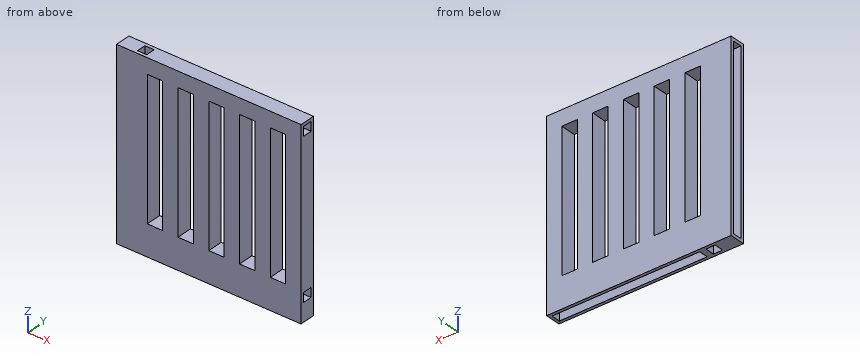
from build123d import *

# Parameters (mm, degrees)
SKETCH3_W           = 152.4
SKETCH3_H           = 152.4
BOSS_EXTRUDE1_DEPTH = 12.7
SKETCH5_W           = 147.32
SKETCH5_H           = 7.62
CUT_EXTRUDE1_DEPTH  = 12.7
SKETCH6_W           = 12.7
SKETCH6_H           = 127
CUT_EXTRUDE3_DEPTH  = 12.7
SKETCH8_W           = 7.62
SKETCH8_H           = 7.62
CUT_EXTRUDE4_DEPTH  = 25.4
SKETCH9_W           = 7.62
SKETCH9_H           = 7.62
CUT_EXTRUDE5_DEPTH  = 25.4
SKETCH10_W          = 7.508888552
SKETCH10_H          = 7.62
CUT_EXTRUDE6_DEPTH  = 25.4
SKETCH11_W          = 7.62
SKETCH11_H          = 7.62
BOSS_EXTRUDE2_DEPTH = 25.4
SKETCH12_W          = 127.135461675
SKETCH12_H          = 12.7
BOSS_EXTRUDE3_DEPTH = 25.4
SKETCH14_W          = 121.92
SKETCH14_H          = 7.62
CUT_EXTRUDE7_DEPTH  = 12.7
SKETCH15_W          = 7.62
SKETCH15_H          = 7.62
CUT_EXTRUDE9_DEPTH  = 25.4


with BuildPart() as part:
    # Sketch3 → Boss-Extrude1 (new body)
    with BuildSketch(Plane(origin=(0, 0, 0), x_dir=(1, 0, 0), z_dir=(0, 1, 0))):
        with Locations((-76.2, 76.2)):
            Rectangle(SKETCH3_W, SKETCH3_H)
    extrude(amount=BOSS_EXTRUDE1_DEPTH)

    # Sketch5 → Cut-Extrude1 (cut)
    with BuildSketch(Plane.ZY.offset(152.4)):
        with Locations((-76.2, 6.35)):
            Rectangle(SKETCH5_W, SKETCH5_H)
    extrude(amount=-CUT_EXTRUDE1_DEPTH, mode=Mode.SUBTRACT)

    # Sketch6 → Cut-Extrude3 (cut)
    with BuildSketch(Plane(origin=(0, 12.7, 0), x_dir=(1, 0, 0), z_dir=(0, 1, 0))):
        with Locations((-120.65, 76.2)):
            Rectangle(SKETCH6_W, SKETCH6_H)
        with Locations((-95.25, 76.2)):
            Rectangle(SKETCH6_W, SKETCH6_H)
        with Locations((-69.85, 76.2)):
            Rectangle(SKETCH6_W, SKETCH6_H)
        with Locations((-44.45, 76.2)):
            Rectangle(SKETCH6_W, SKETCH6_H)
        with Locations((-19.05, 76.2)):
            Rectangle(SKETCH6_W, SKETCH6_H)
    extrude(amount=-CUT_EXTRUDE3_DEPTH, mode=Mode.SUBTRACT)

    # Sketch8 → Cut-Extrude4 (cut)
    with BuildSketch(Plane(origin=(0, 0, 0), x_dir=(0, 0, -1), z_dir=(1, 0, 0))):
        with Locations((146.05, 6.35)):
            Rectangle(SKETCH8_W, SKETCH8_H)
        with Locations((6.35, 6.35)):
            Rectangle(SKETCH8_W, SKETCH8_H)
    extrude(amount=-CUT_EXTRUDE4_DEPTH, mode=Mode.SUBTRACT)

    # Sketch9 → Cut-Extrude5 (cut)
    with BuildSketch(Plane.XY):
        with Locations((-133.35, 6.35)):
            Rectangle(SKETCH9_W, SKETCH9_H)
    extrude(amount=-CUT_EXTRUDE5_DEPTH, mode=Mode.SUBTRACT)

    # Sketch10 → Cut-Extrude6 (cut)
    with BuildSketch(Plane(origin=(0, 0, -152.4), x_dir=(-1, 0, 0), z_dir=(0, 0, -1))):
        with Locations((133.405555724, 6.35)):
            Rectangle(SKETCH10_W, SKETCH10_H)
    extrude(amount=-CUT_EXTRUDE6_DEPTH, mode=Mode.SUBTRACT)

    # Sketch11 → Boss-Extrude2 (add)
    with BuildSketch(Plane(origin=(-25.4, 0, 0), x_dir=(0, 0, -1), z_dir=(1, 0, 0))):
        with Locations((146.05, 6.35)):
            Rectangle(SKETCH11_W, SKETCH11_H)
    extrude(amount=BOSS_EXTRUDE2_DEPTH)

    # Sketch12 → Boss-Extrude3 (add)
    with BuildSketch(Plane(origin=(0, 0, -152.4), x_dir=(-1, 0, 0), z_dir=(0, 0, -1))):
        with Locations((63.567730838, 6.35)):
            Rectangle(SKETCH12_W, SKETCH12_H)
    extrude(amount=-BOSS_EXTRUDE3_DEPTH)

    # Sketch14 → Cut-Extrude7 (cut)
    with BuildSketch(Plane(origin=(0, 0, -152.4), x_dir=(-1, 0, 0), z_dir=(0, 0, -1))):
        with Locations((63.5, 6.35)):
            Rectangle(SKETCH14_W, SKETCH14_H)
    extrude(amount=-CUT_EXTRUDE7_DEPTH, mode=Mode.SUBTRACT)

    # Sketch15 → Cut-Extrude9 (cut)
    with BuildSketch(Plane(origin=(0, 0, 0), x_dir=(0, 0, -1), z_dir=(1, 0, 0))):
        with Locations((133.35, 6.35)):
            Rectangle(SKETCH15_W, SKETCH15_H)
    extrude(amount=-CUT_EXTRUDE9_DEPTH, mode=Mode.SUBTRACT)


solid = part.part
Input: part model. Units: mm. Frame: model coordinates. Round coordinates to 2 decimals unless told otherwise and drop trailing zeros. Order: outer loops, then holes, each group sorted by start corner. A loop starts at its lowest first (then second) coordinate and runs counter-clockwise, first axis right, second up. Notation, with made-up numbers: (-39.75, 68.25) - (-21.75, 68.25) arc R11 ccw to (-21.75, 79.25) - close; hole circle Ø4 at (1, 1). An arc over 180 degrees is marked (long way). Use a Markdown table: item, result.
1. Material intervals for probe 1 along Z at (x, y) = (-14, 7.75); probe 2 along X at (y, z) = (2, -81.5); probe 3 along X at (y, z) = (6.75, -38), sorted ascending.
Evaluation:
| item | result |
|---|---|
| probe 1 | -139.7 to -137.16, -129.54 to -127, -12.7 to -10.16, -2.54 to 0 |
| probe 2 | -152.4 to -127, -114.3 to -101.6, -88.9 to -76.2, -63.5 to -50.8, -38.1 to -25.4, -12.7 to 0 |
| probe 3 | -139.7 to -127, -114.3 to -101.6, -88.9 to -76.2, -63.5 to -50.8, -38.1 to -25.4, -12.7 to 0 |
2. Section A-A on z = -66. Return the cut outline in (x, y).
Evaluation:
| item | result |
|---|---|
| outline | (-152.4, 0) - (-127, 0) - (-127, 12.7) - (-152.4, 12.7) - (-152.4, 10.16) - (-139.7, 10.16) - (-139.7, 2.54) - (-152.4, 2.54) - close; (-114.3, 0) - (-101.6, 0) - (-101.6, 12.7) - (-114.3, 12.7) - close; (-88.9, 0) - (-76.2, 0) - (-76.2, 12.7) - (-88.9, 12.7) - close; (-63.5, 0) - (-50.8, 0) - (-50.8, 12.7) - (-63.5, 12.7) - close; (-38.1, 0) - (-25.4, 0) - (-25.4, 12.7) - (-38.1, 12.7) - close; (-12.7, 0) - (0, 0) - (0, 12.7) - (-12.7, 12.7) - close |
3. Section B-B on x = -41. Return the cut outline in (y, z).
Evaluation:
| item | result |
|---|---|
| outline | (0, -152.4) - (2.54, -152.4) - (2.54, -139.7) - (10.16, -139.7) - (10.16, -152.4) - (12.7, -152.4) - (12.7, -127) - (0, -127) - close; (0, -12.7) - (12.7, -12.7) - (12.7, 0) - (0, 0) - close |
4. First-contact query: pin 1 (1.5 mm diameter, centred on y = 6, z = -33, fed in from -X); pin 2 (2.5 mm diameter, centred on y = 6, z = -134.5, fed in from +X); pin 3 (4 mm diameter, centred on x = -133, y = 5, fed in from +Z). Flat tips, straight axial feed; report the tip coordinate or a pass-through.
Evaluation:
| item | result |
|---|---|
| pin 1 | x = -139.7 |
| pin 2 | x = -25.4 |
| pin 3 | z = -25.4 |
5. Section D-D on y = 6. State how many separate pieces and enclosed holes the cut face has, then the cut area to 3 significant figures.
Evaluation:
| item | result |
|---|---|
| separate pieces | 1 |
| enclosed holes | 5 |
| area | 11,800 mm^2 |
6. Section C-C on x = -141.5. Return the cut outline in (y, z), then the cut area to 3 significant figures.
Evaluation:
| item | result |
|---|---|
| outline | (0, -152.4) - (12.7, -152.4) - (12.7, 0) - (0, 0) - close; hole (2.54, -149.86) - (10.16, -149.86) - (10.16, -2.54) - (2.54, -2.54) - close |
| area | 813 mm^2 |
